Autodesk Inventor part; units mm, degrees
ref_plane "YZ Plane" through (0, 0, 0) normal (1, 0, 0) x (0, 1, 0)
ref_plane "XZ Plane" through (0, 0, 0) normal (0, 1, 0) x (-1, 0, 0)
ref_plane "XY Plane" through (0, 0, 0) normal (0, 0, 1) x (1, 0, 0)
sketch "スケッチ1" plane through (0, 0, 0) normal (0, 1, 0) x (-1, 0, 0)
  circle A0 centre (0, 0) radius 4
  circle A1 centre (0, 0) radius 9.5
  dimension "d0" = 8
  dimension "d1" = 19
extrude "押し出し1" add sketch "スケッチ1" along normal blind 6
sketch "スケッチ2" plane through (0, 6, 0) normal (0, 1, 0) x (1, 0, 0)
  circle A0 centre (0, 0) radius 11
  circle A1 centre (0, 0) radius 9.5
  dimension "d4" = 22
extrude "押し出し2" add sketch "スケッチ2" against normal blind 1.5
fillet "フィレット1" radius 0.3 5 edges at (-11, 6, 0) (-11, 4.5, 0) (9.5, 0, 0) (4, 6, 0) (4, 0, 0)
properties part number "p8-19flange" material "鋼 AISI 1006 85 HR"
For this review, take the finished solid that the model builds, in its own axes (mm). A direction names the side the tool comes from. Give positions to 0.01 mm unless a question says otherwise; leave off trailing zeros. Order: outer loops, then holes, each group sorted by start corner. A loop starts at its lowest first (then second) coordinate and runs counter-clockwise, first axis right, second up. Notation, with made-up numbers: (-16.75, 82.25) - (7.25, 82.25) arc R34 ccw to (7.25, 118.25) - close; hole circle Ø10 at (39, 34.5). An arc over 180 degrees is marked (long way). Answer as a JSON object with one key per item and string values. Group by question number.
Item 1: Take a section at A-A on x = 0. Give the boundary of the cut face in (y, z).
Item 2: Draft analysis for pull direction Z (two halves, no side actions). For faces 1 (the cylindrical face through (-2.38, 5.26, 10.74)), 2 (the cylindrical face through (0.867, 2.962, 3.905)), 3 (the flat face through (0, 4.5, -10)), state which applies: pulls with the +Z half, pulls with the -Z half, needs draft (parallel to the pull), parting line crosses it, or undercut.
Item 3: Take a section at C-C on y = 5.1. Give the boundary of the cut face in (x, z).
Item 4: Machinability: for faces 4 (the flat face through (-2, 0, -4)), 5 (the cylindrical face through (-4.38, 2.37, 8.43)), which of the approach directions +Z, -Z, +X, -X, +Y, -Y give a long, thin tool a straight path to every point of the face, cutting with its end or side? Answer none if there is none.
Item 5: Wall thickness on line 1 along Z through (x, y) = (0, 4.4); line 2 along Z through (x, y) = (0, 4.75); line 3 along X through (y, z) = (5.7, -1.25): over which ranges is each line inside the solid? List them lowest first.
Item 6: Take a section at D-D on y = 0.95. Give the boundary of the cut face in (x, z), and give its area (3 significant figures).
Item 7: Clearance check with flat-ended pins moving along their axes: pin 1 Ø1.5 at (y, z) = (4.5, -2.5) entering from +X; pin 2 Ø3 at (x, y) = (-8.5, 2) entering from +Z; pin 3 Ø3 at (y, z) = (3.5, 8.5) entering from +X. State where each tip first meets the part, or that it passes through.
Item 8: Take a section at B-B on z = 0. Give the boundary of the cut face in (x, y), and give its area (3 significant figures).
Reported:
{
 "1": {"outline": "(0, -9.2) arc R0.3 ccw to (0.3, -9.5) - (4.5, -9.5) - (4.5, -10.7) arc R0.3 ccw to (4.8, -11) - (5.7, -11) arc R0.3 ccw to (6, -10.7) - (6, -4.3) arc R0.3 ccw to (5.7, -4) - (0.3, -4) arc R0.3 ccw to (0, -4.3) - close; (0, 4.3) arc R0.3 ccw to (0.3, 4) - (5.7, 4) arc R0.3 ccw to (6, 4.3) - (6, 10.7) arc R0.3 ccw to (5.7, 11) - (4.8, 11) arc R0.3 ccw to (4.5, 10.7) - (4.5, 9.5) - (0.3, 9.5) arc R0.3 ccw to (0, 9.2) - close"},
 "2": {"face 1": "parting line crosses it", "face 2": "undercut", "face 3": "needs draft"},
 "3": {"outline": "circle Ø22 at (0, 0); hole circle Ø8 at (0, 0)"},
 "4": {"face 4": "+Z, -Z, +X, -X, -Y", "face 5": "-Y"},
 "5": {"line 1": "-9.5 to -4, 4 to 9.5", "line 2": "-11 to -4, 4 to 11", "line 3": "-10.93 to -3.8, 3.8 to 10.93"},
 "6": {"outline": "circle Ø19 at (0, 0); hole circle Ø8 at (0, 0)", "area": "233 mm^2"},
 "7": {"pin 1": "x = 10.85", "pin 2": "z = 6.42", "pin 3": "x = 7.96"},
 "8": {"outline": "(-11, 4.8) arc R0.3 ccw to (-10.7, 4.5) - (-9.5, 4.5) - (-9.5, 0.3) arc R0.3 ccw to (-9.2, 0) - (-4.3, 0) arc R0.3 ccw to (-4, 0.3) - (-4, 5.7) arc R0.3 ccw to (-4.3, 6) - (-10.7, 6) arc R0.3 ccw to (-11, 5.7) - close; (4, 0.3) arc R0.3 ccw to (4.3, 0) - (9.2, 0) arc R0.3 ccw to (9.5, 0.3) - (9.5, 4.5) - (10.7, 4.5) arc R0.3 ccw to (11, 4.8) - (11, 5.7) arc R0.3 ccw to (10.7, 6) - (4.3, 6) arc R0.3 ccw to (4, 5.7) - close", "area": "70.3 mm^2"}
}
